Autodesk Inventor part; units mm, degrees
ref_plane "YZ Plane" through (0, 0, 0) normal (1, 0, 0) x (0, 1, 0)
ref_plane "XZ Plane" through (0, 0, 0) normal (0, 1, 0) x (-1, 0, 0)
ref_plane "XY Plane" through (0, 0, 0) normal (0, 0, 1) x (1, 0, 0)
sketch "Sketch1" plane through (0, 0, 0) normal (0, 0, 1) x (1, 0, 0)
  line L0 (-7.5, 7.5) -> (7.5, 7.5) construction
  line L1 (-7.5, 7.5) -> (-7.5, 3.1) construction
  line L2 (-7.5, 3.1) -> (-5.5, 3.1) construction
  line L3 (-5.5, 5.6) -> (-5.5, 3.1) construction
  line L4 (-5.5, 5.6) -> (-3, 3.1) construction
  line L5 (-3, 0) -> (0, 0)
  line L6 (0, 0) -> (0, 7.5)
  arc A0 (-6.5, 7.5) -> (-7.5, 6.5) centre (-6.5, 6.5) ccw
  line L7 (-7.5, 6.5) -> (-7.5, 3.1) construction
  line L8 (-6.5, 7.5) -> (0, 7.5)
  arc A1 (-4.6464, 4.7464) -> (-5.5, 4.3929) centre (-5, 4.3929) ccw
  line L9 (-5.5, 4.3929) -> (-5.5, 3.1)
  line L10 (-3, 3.1) -> (-3, 0) construction
  arc A2 (-3, 2.8929) -> (-3.1464, 3.2464) centre (-3.5, 2.8929) ccw
  line L11 (-4.6464, 4.7464) -> (-3.1464, 3.2464)
  line L12 (-3, 2.8929) -> (-3, 0)
  line L13 (-7.5, 3.1) -> (-7, 3.1) construction
  line L14 (-7, 3.1) -> (-7, 3.6)
  line L15 (-7, 3.6) -> (-7.5, 3.6)
  line L16 (-7.5, 3.6) -> (-7.5, 3.1) construction
  line L17 (-7.5, 6.5) -> (-7.5, 3.6)
  line L18 (-5.5, 3.1) -> (-7, 3.1)
  dimension "d0" = 15
  dimension "d1" = 7.5
  dimension "d3" = 2
  dimension "d4" = 2.5
  dimension "d5" = 45
  dimension "d9" = 1
  dimension "d10" = 0.5
  dimension "d11" = 0.5
  dimension "d12" = 0.5
  dimension "d13" = 3.1
extrude "Extrusion1" add sketch "Sketch1" against normal blind 1000
mirror "Mirror3" about plane through (0, 0, 0) normal (1, 0, 0) of "Extrusion1"
mirror "Mirror4" about plane through (0, 0, 0) normal (0, 1, 0) of "Extrusion1", "Mirror3"
equation "\"d1\" = 0.5 * d0"
properties part number "profile_0001_0001"
Could you check a few things on this model? Use its own coordinates, in mm. Give positions to 0.01 mm unless a question says otherwise; leave off trailing zeros. Order: outer loops, then holes, each group sorted by start corner. A loop starts at its lowest first (then second) coordinate and runs counter-clockwise, first axis right, second up.
1. I need wall thicknesses on L1, parallel to X at y = -3.75, z = -956; L2, parallel to Y at x = -3.5, z = -374; L3, parallel to Y at x = 4.5, z = -424.5. Which ranges of each line are inside material? Lowest first, please.
2. Suppose I cut it at A-A (y = 0). List the corners of the cut face in (x, z) for me, plus the area to 3 significant figures.
3. Will these pins go through, and if not, where does the flat tip stop? P1, Ø0.6, axis at x = -7.5, z = -457, coming from the +Y side; P2, Ø3, axis at y = -0.5, z = -415.5, coming from the +X side; P3, Ø2, axis at y = -0.5, z = -729, coming from the -X side.
Solved:
1. L1: x = -7.5 to -5.5, -3.65 to 3.65, 5.5 to 7.5
1. L2: y = -7.5 to -3.6, 3.6 to 7.5
1. L3: y = -7.5 to -4.6, 4.6 to 7.5
2. outline: (-3, -1000) - (3, -1000) - (3, 0) - (-3, 0) - close
2. area: 6,000 mm2
3. P1: stops at y = 7.21
3. P2: stops at x = 3
3. P3: stops at x = -3
